Design review of the part built by this model. Coordinates are the model's own, in mm. A direction names the side the tool comes from. Coordinates: 2 decimals unless noted, no trailing zeros. Write each loop counter-clockwise with the first axis right and the second up, starting at its lowest first coordinate (ties: lowest second). Pieces come first, ordered by that corner, then holes.
Q1. Add section B-B, the plane y = 35.5. Give the boundary of the cut face in (x, z), plus the area to 3 significant figures.
Q2. Add section C-C, the plane z = 17. Give the boundary of the cut face in (x, y).
Q3. To check wall thickness, follow probe 1 along Z at (x, y) = (-20, 10.25); probe 2 along Z at (x, y) = (-6, 20); probe 3 along Z at (x, y) = (-11, 28.5). State the ranges of each line that lie inside material, in increasing order.
Q4. Add section A-A, the plane x = -30. Give the number of separate pieces and of enclosed holes in the cut face, plus the area to 3 significant figures.
Q5. The part is to be moulded in two halves that separate along Z. For faces 1 (the face through (-32, 20, 22)), 2 (the face through (-27.854, 8.176, 55.028)), 3 (the face through (-5, 30, 53)), say which applies: +Z half, -Z half, draft (parallel to the pull), parting line (faces both ways), or undercut.
Q6. Machinability: for faces 4 (the face through (-22, 33, 20)), 5 (the face through (-9.748, 30.099, 55.028)), 6 (the face through (-22, 11, 25)), 7 (the face through (-11, 20, 2)), which of the approach directions +Z, -Z, +X, -X, +Y, -Y give a long, thin tool a straight path to every point of the face, cutting with its end or side? Answer none if there is none.
Q7. Clearance check with flat-ended pins moving along their axes: pin 1 Ø20 at (y, z) = (21, 37) entering from -X; pin 2 Ø1 at (y, z) = (25.5, 38) entering from -X; pin 3 Ø2.5 at (x, z) = (-19, 47) entering from +Y. State where each tip first meets the part, or that it passes through.
from build123d import *

# Parameters (mm, degrees)
ESQUISSE1_W              = 40
ESQUISSE1_H              = 40
BOSS_EXTRU_1_DEPTH       = 50
ESQUISSE2_R              = 5
ENL_V_MAT_EXTRU_1_DEPTH  = 41
ESQUISSE3_R              = 5
ENL_V_MAT_EXTRU_2_DEPTH  = 41
ESQUISSE4_W              = 22
ESQUISSE4_H              = 14
ENL_V_MAT_EXTRU_3_DEPTH  = 29
ESQUISSE5_W              = 14
ESQUISSE5_H              = 20
ENL_V_MAT_EXTRU_4_DEPTH  = 29
ESQUISSE6_W              = 20
ESQUISSE6_H              = 14
ENL_V_MAT_EXTRU_5_DEPTH  = 24
ESQUISSE7_W              = 14
ESQUISSE7_H              = 22
ENL_V_MAT_EXTRU_6_DEPTH  = 24
ESQUISSE10_R             = 11
ENL_V_MAT_EXTRU_9_DEPTH  = 7
ESQUISSE11_R             = 12.5
ENL_V_MAT_EXTRU_10_DEPTH = 1.5
ESQUISSE14_R             = 11
ENL_V_MAT_EXTRU_11_DEPTH = 7
ESQUISSE15_R             = 12.5
ENL_V_MAT_EXTRU_12_DEPTH = 1.5
ESQUISSE16_W             = 40
ESQUISSE16_H             = 40
BOSS_EXTRU_2_DEPTH       = 7
ESQUISSE17_R             = 2.25
ENL_V_MAT_EXTRU_13_DEPTH = 15
ESQUISSE18_W             = 7
ESQUISSE18_H             = 3
ENL_V_MAT_EXTRU_14_DEPTH = 12
ESQUISSE19_W             = 3
ESQUISSE19_H             = 7
ENL_V_MAT_EXTRU_15_DEPTH = 12


with BuildPart() as part:
    # Esquisse1 → Boss.-Extru.1 (new body)
    with BuildSketch(Plane.XY):
        with Locations((-20, 20)):
            Rectangle(ESQUISSE1_W, ESQUISSE1_H)
    extrude(amount=BOSS_EXTRU_1_DEPTH)

    # Esquisse2 → Enlèv. mat.-Extru.1 (cut, through all)
    with BuildSketch(Plane(origin=(0, 40, 0), x_dir=(1, 0, 0), z_dir=(0, 1, 0))):
        with Locations(Location((-20, -15, 0), (0, 0, 270))):  # turned: the seam where the file's is
            Circle(ESQUISSE2_R)
    extrude(amount=-ENL_V_MAT_EXTRU_1_DEPTH, mode=Mode.SUBTRACT)

    # Esquisse3 → Enlèv. mat.-Extru.2 (cut, through all)
    with BuildSketch(Plane.ZY.offset(40)):
        with Locations((35, 20)):
            Circle(ESQUISSE3_R)
    extrude(amount=-ENL_V_MAT_EXTRU_2_DEPTH, mode=Mode.SUBTRACT)

    # Esquisse4 → Enlèv. mat.-Extru.3 (cut)
    with BuildSketch(Plane.ZY.offset(40)):
        with Locations((11, 20)):
            Rectangle(ESQUISSE4_W, ESQUISSE4_H)
    extrude(amount=-ENL_V_MAT_EXTRU_3_DEPTH, mode=Mode.SUBTRACT)

    # Esquisse5 → Enlèv. mat.-Extru.4 (cut)
    with BuildSketch(Plane.XZ):
        with Locations((-20, 35)):
            Rectangle(ESQUISSE5_W, ESQUISSE5_H)
    extrude(amount=-ENL_V_MAT_EXTRU_4_DEPTH, mode=Mode.SUBTRACT)

    # Esquisse6 → Enlèv. mat.-Extru.5 (cut)
    with BuildSketch(Plane(origin=(0, 0, 0), x_dir=(0, 0, -1), z_dir=(1, 0, 0))):
        with Locations((-15, 20)):
            Rectangle(ESQUISSE6_W, ESQUISSE6_H)
    extrude(amount=-ENL_V_MAT_EXTRU_5_DEPTH, mode=Mode.SUBTRACT)

    # Esquisse7 → Enlèv. mat.-Extru.6 (cut)
    with BuildSketch(Plane(origin=(0, 40, 0), x_dir=(1, 0, 0), z_dir=(0, 1, 0))):
        with Locations((-20, -39)):
            Rectangle(ESQUISSE7_W, ESQUISSE7_H)
    extrude(amount=-ENL_V_MAT_EXTRU_6_DEPTH, mode=Mode.SUBTRACT)

    # Esquisse10 → Enlèv. mat.-Extru.9 (cut)
    with BuildSketch(Plane(origin=(0, 40, 0), x_dir=(1, 0, 0), z_dir=(0, 1, 0))):
        with Locations(Location((-20, -15, 0), (0, 0, 270))):  # turned: the seam where the file's is
            Circle(ESQUISSE10_R)
    extrude(amount=-ENL_V_MAT_EXTRU_9_DEPTH, mode=Mode.SUBTRACT)

    # Esquisse11 → Enlèv. mat.-Extru.10 (cut)
    with BuildSketch(Plane(origin=(0, 40, 0), x_dir=(1, 0, 0), z_dir=(0, 1, 0))):
        with Locations(Location((-20, -15, 0), (0, 0, 270))):  # turned: the seam where the file's is
            Circle(ESQUISSE11_R)
    extrude(amount=-ENL_V_MAT_EXTRU_10_DEPTH, mode=Mode.SUBTRACT)

    # Esquisse14 → Enlèv. mat.-Extru.11 (cut)
    with BuildSketch(Plane.ZY.offset(40)):
        with Locations((35, 20)):
            Circle(ESQUISSE14_R)
    extrude(amount=-ENL_V_MAT_EXTRU_11_DEPTH, mode=Mode.SUBTRACT)

    # Esquisse15 → Enlèv. mat.-Extru.12 (cut)
    with BuildSketch(Plane.ZY.offset(40)):
        with Locations((35, 20)):
            Circle(ESQUISSE15_R)
    extrude(amount=-ENL_V_MAT_EXTRU_12_DEPTH, mode=Mode.SUBTRACT)

    # Esquisse16 → Boss.-Extru.2 (add)
    with BuildSketch(Plane.XY.offset(50)):
        with Locations((-20, 20)):
            Rectangle(ESQUISSE16_W, ESQUISSE16_H)
    extrude(amount=BOSS_EXTRU_2_DEPTH)

    # Esquisse17 → Enlèv. mat.-Extru.13 (cut)
    with BuildSketch(Plane.XY.offset(57)):
        with Locations((-30, 7.5)):
            Circle(ESQUISSE17_R)
        with Locations((-7.5, 30)):
            Circle(ESQUISSE17_R)
    extrude(amount=-ENL_V_MAT_EXTRU_13_DEPTH, mode=Mode.SUBTRACT)

    # Esquisse18 → Enlèv. mat.-Extru.14 (cut)
    with BuildSketch(Plane.XZ):
        with Locations((-30, 51.5)):
            Rectangle(ESQUISSE18_W, ESQUISSE18_H)
    extrude(amount=-ENL_V_MAT_EXTRU_14_DEPTH, mode=Mode.SUBTRACT)

    # Esquisse19 → Enlèv. mat.-Extru.15 (cut)
    with BuildSketch(Plane(origin=(0, 0, 0), x_dir=(0, 0, -1), z_dir=(1, 0, 0))):
        with Locations((-51.5, 30)):
            Rectangle(ESQUISSE19_W, ESQUISSE19_H)
    extrude(amount=-ENL_V_MAT_EXTRU_15_DEPTH, mode=Mode.SUBTRACT)


solid = part.part
Here are the results:
1. outline: (-40, 0) - (0, 0) - (0, 57) - (-40, 57) - close; hole circle Ø22 at (-20, 15); hole (-27, 28) - (-13, 28) - (-13, 50) - (-27, 50) - close
1. area: 1,590 mm2
2. outline: (-40, 0) - (-24.58, 0) - (-24.58, 13) - (-40, 13) - close; (-40, 27) - (-24.58, 27) - (-24.58, 33) - (-30.82, 33) - (-30.82, 38.5) - (-32.34, 38.5) - (-32.34, 40) - (-40, 40) - close; (-15.42, 0) - (0, 0) - (0, 13) - (-15.42, 13) - close; (-15.42, 27) - (0, 27) - (0, 40) - (-7.66, 40) - (-7.66, 38.5) - (-9.18, 38.5) - (-9.18, 33) - (-15.42, 33) - close
3. probe 1: z = 0 to 10, 20 to 25, 45 to 57
3. probe 2: z = 0 to 5, 25 to 30, 40 to 57
3. probe 3: z = 0 to 50, 53 to 57
4. separate pieces: 2
4. enclosed holes: 1
4. area: 1,730 mm2
5. face 1: -Z half
5. face 2: draft
5. face 3: undercut
6. face 4: +Y
6. face 5: +Z
6. face 6: -Y
6. face 7: -Z, -X
7. pin 1: stops at x = -38.5
7. pin 2: stops at x = -33
7. pin 3: stops at y = 16
